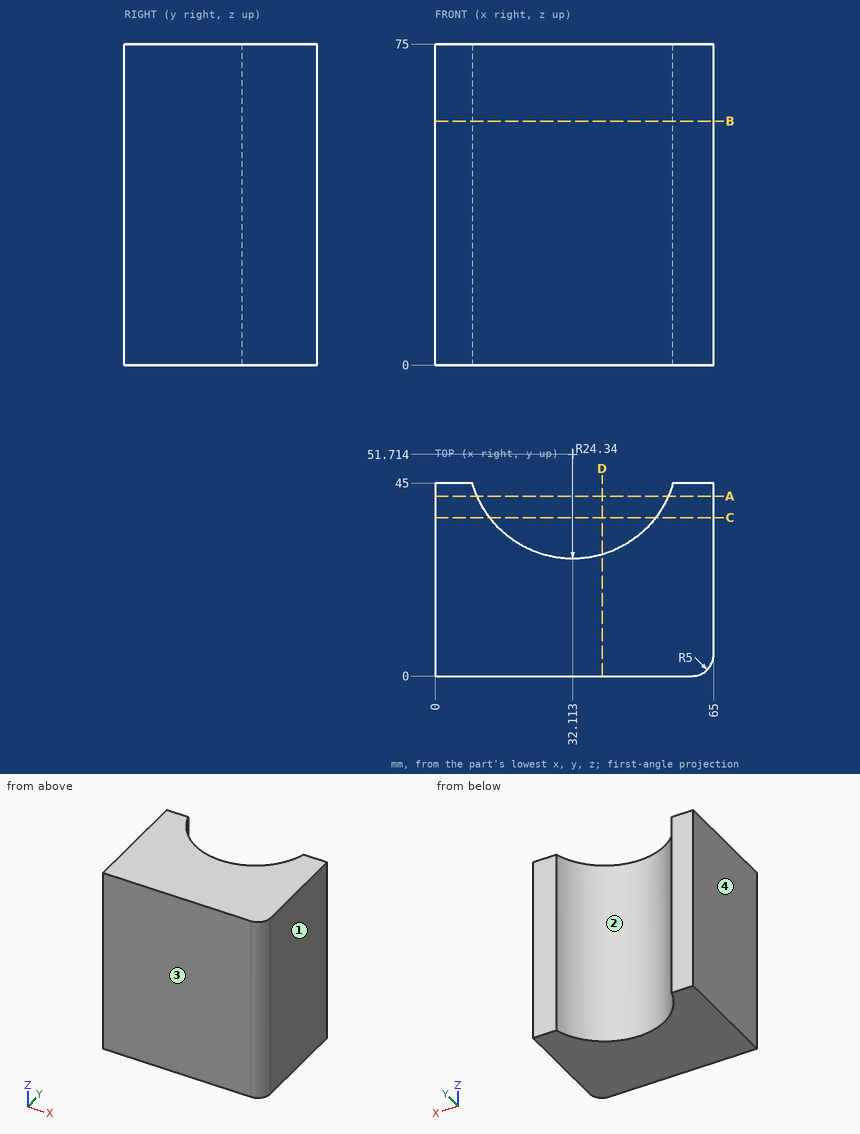
The drawing under review shows one solid part. Ordinate dimensions are in mm from its lowest x, y, z. Round coordinates to 2 decimals unless told otherwise and drop trailing zeros. Write each loop counter-clockwise with the first axis right and the second up, starting at its lowest first coordinate (ties: lowest second). Pieces come first, ordered by that corner, then holes. Notation, with made-up numbers: (75.5, -36) - (98.5, -36) arc R19 ccw to (98.5, -31) - close; hole circle Ø9 at (23.25, -7). An arc over 180 degrees is marked (long way). Use a Markdown table: item, result. Add a question column.
1. We need section C-C (y = 37). State the section outline as (x, z) points.
2. Clearance check with a flat-ended pin moving along its axis: pin 1 (3 mm diameter, centred on x = 24, z = 9, fed in from -Y). State where the tip first meets the part, or that it passes through.
3. Mouldability with a two-part tool opening along X and no side actions: class the marked faces 1, 2, 3 and 4 as +X half, -X half, draft (parallel to the pull), parting line (faces both ways), or undercut.
4. We need section D-D (x = 39). State the section outline as (y, z) points, then the cut area to 3 significant figures.
5. We need section B-B (z = 57). State the section outline as (x, y) points.
6. We need section A-A (y = 42). State the section outline as (x, z) points (1 decimal).
7. Wall thickness on probe 1 along X at (y, z) = (41.5, 10.5); probe 2 along X at (y, z) = (35, 62); probe 3 along X at (y, z) = (4.5, 6) (1 decimal): over which ranges is each line inside the solid? List them lowest first.
Output:
| question | item | result |
|---|---|---|
| 1 | outline | (0, 0) - (12.72, 0) - (12.72, 75) - (0, 75) - close; (51.5, 0) - (65, 0) - (65, 75) - (51.5, 75) - close |
| 2 | pin 1 | stops at y = 0 |
| 3 | face 1 | +X half |
| 3 | face 2 | undercut |
| 3 | face 3 | draft |
| 3 | face 4 | -X half |
| 4 | outline | (0, 0) - (28.37, 0) - (28.37, 75) - (0, 75) - close |
| 4 | area | 2,130 mm2 |
| 5 | outline | (0, 0) - (60, 0) arc R5 ccw to (65, 5) - (65, 45) - (55.51, 45) arc R24.34 cw to (8.72, 45) - (0, 45) - close |
| 6 | outline | (0, 0) - (9.8, 0) - (9.8, 75) - (0, 75) - close; (54.4, 0) - (65, 0) - (65, 75) - (54.4, 75) - close |
| 7 | probe 1 | x = 0 to 10.02, 54.21 to 65 |
| 7 | probe 2 | x = 0 to 14.42, 49.81 to 65 |
| 7 | probe 3 | x = 0 to 65 |
